```python
from build123d import *

# Parameters (mm, degrees)
F1_W     = 83.82
F1_H     = 38.1
F1_R     = 3.175
F1_R_2   = 1.651
F2_DEPTH = 2.54
F3_DEPTH = 10.16
F4_R     = 5.08


with BuildPart() as f2:
    # F1 (on Top) → F2 (new body)
    with BuildSketch(Plane.XY):
        Rectangle(F1_W, F1_H)
        with Locations((-37.4015, -15.5575)):
            Circle(F1_R, mode=Mode.SUBTRACT)
        with Locations((37.4015, -15.5575)):
            Circle(F1_R, mode=Mode.SUBTRACT)
        with Locations((-37.4015, 15.5575)):
            Circle(F1_R, mode=Mode.SUBTRACT)
        with Locations((37.4015, 15.5575)):
            Circle(F1_R, mode=Mode.SUBTRACT)
        with Locations((-37.4015, 15.5575)):
            Circle(F1_R)
        with Locations((-37.4015, 15.5575)):
            Circle(F1_R_2, mode=Mode.SUBTRACT)
        with Locations((37.4015, -15.5575)):
            Circle(F1_R)
        with Locations((37.4015, -15.5575)):
            Circle(F1_R_2, mode=Mode.SUBTRACT)
        with Locations((37.4015, 15.5575)):
            Circle(F1_R)
        with Locations((37.4015, 15.5575)):
            Circle(F1_R_2, mode=Mode.SUBTRACT)
        with Locations((-37.4015, -15.5575)):
            Circle(F1_R)
        with Locations((-37.4015, -15.5575)):
            Circle(F1_R_2, mode=Mode.SUBTRACT)
        with Locations((37.4015, 15.5575)):
            Circle(F1_R_2)
        with Locations((-37.4015, 15.5575)):
            Circle(F1_R_2)
        with Locations((-37.4015, -15.5575)):
            Circle(F1_R_2)
        with Locations((37.4015, -15.5575)):
            Circle(F1_R_2)
    extrude(amount=-F2_DEPTH)

    # F1 (on Top) → F3 (join)
    with BuildSketch(Plane.XY):
        with Locations((-37.4015, -15.5575)):
            Circle(F1_R)
        with Locations((-37.4015, -15.5575)):
            Circle(F1_R_2, mode=Mode.SUBTRACT)
        with Locations((-37.4015, 15.5575)):
            Circle(F1_R)
        with Locations((-37.4015, 15.5575)):
            Circle(F1_R_2, mode=Mode.SUBTRACT)
        with Locations((37.4015, -15.5575)):
            Circle(F1_R)
        with Locations((37.4015, -15.5575)):
            Circle(F1_R_2, mode=Mode.SUBTRACT)
        with Locations((37.4015, 15.5575)):
            Circle(F1_R)
        with Locations((37.4015, 15.5575)):
            Circle(F1_R_2, mode=Mode.SUBTRACT)
    extrude(amount=F3_DEPTH)

    # F4
    f4_edges = [f2.edges().sort_by_distance(p)[0] for p in [
        (-41.91, -19.05, -1.27),
        (41.91, -19.05, -1.27),
        (41.91, 19.05, -1.27),
        (-41.91, 19.05, -1.27),
    ]]
    fillet(f4_edges, radius=F4_R)


solid = f2.part
```
Model file for the job. Use its own axes, mm. A direction names the side the tool comes from. Coordinates: 2 decimals unless noted, no trailing zeros. Order: outer loops, then holes, each group sorted by start corner. A loop starts at its lowest first (then second) coordinate and runs counter-clockwise, first axis right, second up. Notation, with made-up numbers: (50.25, -11) -> (92.25, -11) arc R21 cw to (92.25, 21) -> close; hole circle Ø1 at (-27, 32.25). An arc over 180 degrees is marked (long way). Answer as a JSON object with one key per item and string values. Group by question number.
1) Pull direction Y, two halves, no side cores. Call faces 3 (the face through (-40.461, 17.522, -1.288)), 4 (the face through (-1, 0, -2.54)), 5 (the face through (-35.876, -16.19, 5.009)): +Y half, -Y half, draft (parallel to the pull), parting line (faces both ways), or undercut.
2) Which spindle directions (+Z, -Z, +X, -X, +Y, -Y) get a long thin tool onto all of the face, cutting with end or side? Do faces 1 (the face through (35.06, 17.7, 5.01)), 2 (the face through (-36, -17, 10.16)). Say none if no direction does.
3) Drill centre lines: L1, parallel to X at y = -15, z = 1.5; L2, parallel to Z at x = -12.5, y = 13.5; L3, parallel to X at y = 17, z = 9.75. Where is each one in solid material? Low to high.
4) Cut at A-A, the plane z = 9.25. Count the separate pieces of the cut face and the enclosed holes in it, then the cut area to 3 significant figures.
5) Cut at C-C, the plane x = -1.5. Write the cut outline in (y, z), then the cut area to 3 significant figures.
6) Flat gauge pins, fed straight in: pin 1 (1 mm diameter, centred on y = 15, z = 4.5, fed in from -X); pin 2 (19 mm diameter, centred on x = 11, y = 6.5, fed in from +Z); pin 3 (1.5 mm diameter, centred on y = -12.5, z = 5.5, fed in from -X). Where does each tip first touch, or does it go through?
7) Cut at B-B, the plane y = 7.5. Write the cut outline in (x, z).
Check values:
{
 "1": {"face 3": "+Y half", "face 4": "draft", "face 5": "undercut"},
 "2": {"face 1": "+Z", "face 2": "+Z, +X, -X, +Y, -Y"},
 "3": {"L1": "x = -40.53 to -38.96, -35.85 to -34.28, 34.28 to 35.85, 38.96 to 40.53", "L2": "z = -2.54 to 0", "L3": "x = -40.23 to -38.2, -36.6 to -34.57, 34.57 to 36.6, 38.2 to 40.23"},
 "4": {"separate pieces": "4", "enclosed holes": "4", "area": "92.4 mm²"},
 "5": {"outline": "(-19.05, -2.54) -> (19.05, -2.54) -> (19.05, 0) -> (-19.05, 0) -> close", "area": "96.8 mm²"},
 "6": {"pin 1": "stops at x = -40.58", "pin 2": "stops at z = 0", "pin 3": "stops at x = -39.58"},
 "7": {"outline": "(-41.91, -2.54) -> (41.91, -2.54) -> (41.91, 0) -> (-41.91, 0) -> close"}
}
